Geometry check sheet. Reference: the model listing, model coordinates, mm. Face numbers are marked on the shaded views. A direction names the side the tool comes from. Round coordinates to 2 decimals unless told otherwise and drop trailing zeros. Order: outer loops, then holes, each group sorted by start corner. A loop starts at its lowest first (then second) coordinate and runs counter-clockwise, first axis right, second up.
(1) Sectioned sample at A-A (y = -9.5). Record the boundary of the cut face in (x, z), plus the area to 3 significant figures.
(2) Sectioned sample at C-C (x = -108.5). Record the boundary of the cut face in (y, z) (3 decimals).
(3) Go/stop test with flat-tipped pins: pin 1 (11 mm diameter, centred on x = 0, z = 0, fed in from +Y); pin 2 (1 mm diameter, centred on x = -41, y = -11.5, fed in from +Z); pin 3 (5 mm diameter, centred on x = -26, z = -32.5, fed in from -Y); pin 4 (1 mm diameter, centred on x = -16.5, y = -7, fed in from +Z). Record where each tip stops, or that it passes through.
(4) Material ranges on line 1 along Y through (x, z) = (-65, -52); line 2 along Z through (x, y) = (0, -6); line 3 along Z through (x, y) = (-18.5, -12.5), recorded low to high.
(5) Sectioned sample at B-B (x = 0). Record the boundary of the cut face in (y, z) (3 decimals).
(6) Set-up check for the marked faces 1 and 2: record each of +Z, -Z, +X, -X, +Y, -Y from which the full face is reachable in a straight line by a thin tool's end or side.
(7) Sectioned sample at D-D (z = -10). Record the boundary of the cut face in (x, y) (3 decimals), plus the area to 3 significant figures.
from build123d import *

# Parameters (mm, degrees)
F0_R     = 4.2291
F1_DEPTH = 15.875
F3_DEPTH = 10.3124


# Not quite as in the source:
# - a feature of the source that left no trace in its solid (it failed there, or was rolled back) is left out


with BuildPart() as f1:
    # F0 (on Front) → F1 (new body)
    with BuildSketch(Plane.XZ):
        with BuildLine():
            Line((14.3947540456, 8.4944370214), (-39.560838545, 15.1193507659))
            Line((-39.560838545, 15.1193507659), (-58.5532654186, -14.1264219546))
            ThreePointArc((-58.5532654186, -14.1264219546), (-64.8424818087, -20.1998476249), (-73.1576066321, -22.9015954566))
            Line((-73.1576066321, -22.9015954566), (-155.5821148258, -30.1128055203))
            Line((-155.5821148258, -30.1128055203), (-137.3697370291, -80.1509022713))
            Line((-137.3697370291, -80.1509022713), (-23.2329600585, -80.1509022713))
            Line((-23.2329600585, -80.1509022713), (14.3947540456, 8.4944370214))
        make_face()
        with Locations((-34.7655170351, 4.2686687437)):
            Circle(F0_R, mode=Mode.SUBTRACT)
        Circle(F0_R, mode=Mode.SUBTRACT)
    extrude(amount=F1_DEPTH)

    # F2 (on face) → F3 (cut)
    with BuildSketch(Plane.XZ.offset(15.875)):
        with BuildLine():
            Line((-8.0578011567, -23.7078415676), (-153.2887042884, -36.4138991852))
            Line((-153.2887042884, -36.4138991852), (-137.3697370291, -80.1509022713))
            Line((-137.3697370291, -80.1509022713), (-23.2329600585, -80.1509022713))
            Line((-23.2329600585, -80.1509022713), (4.6424392905, -14.4805767668))
            ThreePointArc((4.6424392905, -14.4805767668), (-0.4282074312, -20.8552533629), (-8.0578011567, -23.7078415676))
        make_face()
    extrude(amount=-F3_DEPTH, mode=Mode.SUBTRACT)


solid = f1.part
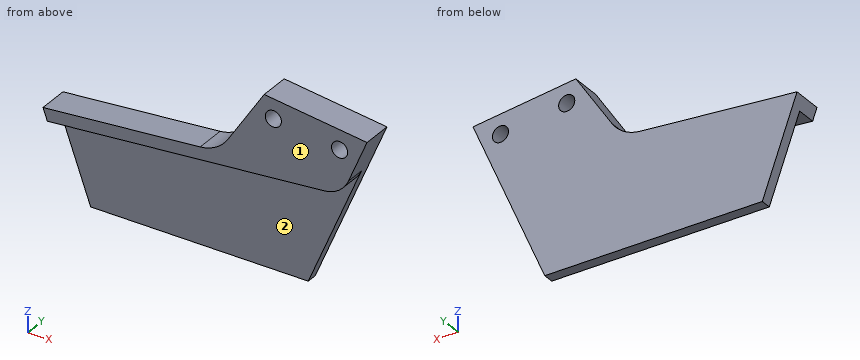
Answer below:
1. outline: (-155.58, -30.11) - (-153.29, -36.41) - (-8.06, -23.71) arc R15.24 ccw to (4.64, -14.48) - (14.39, 8.49) - (-39.56, 15.12) - (-58.55, -14.13) arc R19.43 cw to (-73.16, -22.9) - close; hole circle Ø8.46 at (-34.77, 4.27); hole circle Ø8.46 at (0, 0)
1. area: 2,790 mm2
2. outline: (-15.875, -32.495) - (-5.563, -32.495) - (-5.563, -80.151) - (0, -80.151) - (0, -25.994) - (-15.875, -25.994) - close
3. pin 1: stops at y = 0
3. pin 2: stops at z = 13.67
3. pin 3: stops at y = -5.56
3. pin 4: stops at z = 12.35
4. line 1: y = -5.56 to 0
4. line 2: z = -20.53 to -4.23, 4.23 to 10.26
4. line 3: z = -24.62 to 12.53
5. outline: (-15.875, -20.532) - (-5.563, -20.532) - (-5.563, -25.417) - (0, -25.417) - (0, -4.229) - (-15.875, -4.229) - close; (-15.875, 4.229) - (0, 4.229) - (0, 10.262) - (-15.875, 10.262) - close
6. face 1: +Z, -Z, +X, -X, -Y
6. face 2: -Z, +X, -Y
7. outline: (-55.874, -15.875) - (6.544, -15.875) - (6.544, 0) - (-55.874, 0) - close
7. area: 991 mm2
